Autodesk Inventor part; units mm, degrees
ref_plane "YZ Plane" through (0, 0, 0) normal (1, 0, 0) x (0, 1, 0)
ref_plane "XZ Plane" through (0, 0, 0) normal (0, 1, 0) x (-1, 0, 0)
ref_plane "XY Plane" through (0, 0, 0) normal (0, 0, 1) x (1, 0, 0)
sketch "Sketch1" plane through (0, 0, 0) normal (1, 0, 0) x (0, 1, 0)
  line L0 (45.5354, 147.0574) -> (-5.2646, 147.0574)
  line L1 (-5.2646, 147.0574) -> (-5.2646, 58.1574)
  arc A0 (-5.2646, 58.1574) -> (45.5354, 58.1574) centre (20.1354, 70.5399) ccw
  line L2 (45.5354, 147.0574) -> (45.5354, 58.1574)
  point P0 (20.1354, 42.2824)
  dimension "d0" = 50.8
  dimension "d1" = 88.9
  dimension "d2" = 15.875
extrude "Extrusion1" add sketch "Sketch1" along normal blind 3.175
sketch "Sketch2" plane through (3.175, 0, 0) normal (1, 0, 0) x (0, 0, -1)
  line L0 (-147.0574, 45.5354) -> (-147.0574, -5.2646)
  line L1 (-82.4462, 40.7576) -> (-58.6337, -0.4869)
  point P0 (-82.4462, 40.7576)
  point P1 (-94.3524, 20.1354)
  point P2 (-58.6337, 40.7576)
  point P3 (-46.7274, 20.1354)
  point P4 (-58.6337, -0.4869)
  point P5 (-82.4462, -0.4869)
  dimension "d5" = 47.625
  dimension "d6" = 30
hole "Hole1" at (3.175, 40.7576, 82.4462) at (3.175, 20.1354, 94.3524) at (3.175, 40.7576, 58.6337) at (3.175, 20.1354, 46.7274) at (3.175, -0.4869, 58.6337) at (3.175, -0.4869, 82.4462) direction (-1, 0, 0) diameter 5.08 end through all
sketch "Sketch3" plane through (3.175, 0, 0) normal (1, 0, 0) x (0, 0, -1)
  line L0 (-147.0574, 45.5354) -> (-147.0574, -5.2646)
  line L1 (-58.1574, 45.5354) -> (-147.0574, 45.5354)
  point P0 (-131.1824, 32.8354)
  point P1 (-131.1824, 7.4354)
  dimension "d18" = 25.4
  dimension "d19" = 12.7
  dimension "d20" = 15.875
hole "Hole2" at (3.175, 32.8354, 131.1824) at (3.175, 7.4354, 131.1824) direction (-1, 0, 0) diameter 6.35 end through all
properties part number "Hub Mount Plate"
The listing builds one solid part. Answer for the finished solid, in the listing's coordinates (mm). Round coordinates to 2 decimals unless told otherwise and drop trailing zeros. Write each loop counter-clockwise with the first axis right and the second up, starting at its lowest first coordinate (ties: lowest second). Pieces come first, ordered by that corner, then holes. Notation, with made-up numbers: (-7.5, 70.5) - (11.5, 70.5) arc R18 ccw to (11.5, 103.5) - close; hole circle Ø10 at (-16, 33). An arc over 180 degrees is marked (long way). Use a Markdown table: item, result. Add a question column.
1. For a pull along Y with two mould halves and no side action, classify faces 1 (the face through (1.565, 5.29, 133.523)), 2 (the face through (2, 45.535, 103)), 3 (the face through (2, 20, 147.057)) as +Y half, -Y half, draft (parallel to the pull), parting line (faces both ways), or undercut.
2. The part is cut by section D-D (z = 82.5). Write down the section's boundary in (x, y) (3 decimals), and give its area (3 significant figures).
3. The part is cut by section B-B (y = 42). Write down the section's boundary in (x, z) (3 decimals).
4. Consider line 1 (Z direction, x = 3, y = 20); line 2 (Z direction, x = 1.4, y = 19.5); line 3 (Y direction, x = 0.8, z = 83.5). Determine where each line is inside the solid, lowest interval first.
5. A flat-ended cylindrical pin translates along its axis: P1, Ø4, axis at y = 40.76, z = 58.63, coming from the +X side. Find the tip coordinate at first contact, or state that the pin passes through.
6. The part is cut by section C-C (x = 1.9). Give the number of separate pieces and of enclosed holes in the cut face, and give its area (3 significant figures).
7. The part is cut by section A-A (z = 93). Write down the section's boundary in (x, y) (3 decimals), and give its area (3 significant figures).
Reported:
| question | item | result |
|---|---|---|
| 1 | face 1 | undercut |
| 1 | face 2 | +Y half |
| 1 | face 3 | draft |
| 2 | outline | (0, -5.265) - (3.175, -5.265) - (3.175, -3.026) - (0, -3.026) - close; (0, 2.053) - (3.175, 2.053) - (3.175, 38.218) - (0, 38.218) - close; (0, 43.297) - (3.175, 43.297) - (3.175, 45.535) - (0, 45.535) - close |
| 2 | area | 129 mm^2 |
| 3 | outline | (0, 52.639) - (3.175, 52.639) - (3.175, 56.418) - (0, 56.418) - close; (0, 60.849) - (3.175, 60.849) - (3.175, 80.231) - (0, 80.231) - close; (0, 84.662) - (3.175, 84.662) - (3.175, 147.057) - (0, 147.057) - close |
| 4 | line 1 | 42.28 to 44.19, 49.26 to 91.82, 96.89 to 147.06 |
| 4 | line 2 | 42.29 to 44.27, 49.19 to 91.89, 96.81 to 147.06 |
| 4 | line 3 | -5.26 to -2.8, 1.82 to 38.45, 43.07 to 45.54 |
| 5 | P1 | through |
| 6 | separate pieces | 1 |
| 6 | enclosed holes | 8 |
| 6 | area | 4,910 mm^2 |
| 7 | outline | (0, -5.265) - (3.175, -5.265) - (3.175, 17.985) - (0, 17.985) - close; (0, 22.285) - (3.175, 22.285) - (3.175, 45.535) - (0, 45.535) - close |
| 7 | area | 148 mm^2 |
